Check sheet for the modelled part. Datum: model origin and axes. Units: mm. A direction names the side the tool comes from. Coordinates: 2 decimals unless noted, no trailing zeros. Loops run counter-clockwise (first coordinate to the right, second up) from the corner with the lowest first, then second, coordinate; pieces in that order, holes last. Notation, with made-up numbers: (84.25, -35.5) - (96.25, -35.5) arc R5 cw to (96.25, -30.5) - close; hole circle Ø3 at (40.25, -8). An arc over 180 degrees is marked (long way). Use a Markdown table: item, result. Add a question column.
1) Tool access check on faces 1 (the flat face through (-4, 16, 4)), 2 (the flat face through (6, 6.29, -2)), 3 (the flat face through (-3.537, 16.247, -3.484)), 4 (the flat face through (-4.24, 16.25, -2.71)). Record the directions out of +Z, -Z, +X, -X, +Y, -Y that give a thin tool (end or side, any length) a straight path to the whole face; none if there is none.
2) Go/stop test with flat-tipped pins: P1, Ø1.5, axis at x = -3, z = -6, coming from the +Y side; P2, Ø3, axis at y = 11, z = -1.5, coming from the +X side; P3, Ø2, axis at x = 3.5, y = 9, coming from the -Z side. Record where each tip stops, or that it passes through.
3) Sectioned sample at A-A, the plane z = 0. Enter the section's corners in (x, y).
4) Thickness scan on line 1 (Y direction, x = 5.75, z = 4); line 2 (X direction, y = 4.75, z = 0); line 3 (X direction, y = 7, z = 0). Record the ranges inside material, lowest first.
5) Sectioned sample at B-B, the plane y = 7. Enter the section's corners in (x, z).
6) Draft check along Z on faces 5 (the flat face through (-4.765, 16.247, 1.627)), 6 (the flat face through (0, 0, 3)), 7 (the cylindrical face through (1.802, 10.234, 5.723)). Enter one of: pulls with the +Z half, pulls with the -Z half, needs draft (parallel to the pull), parting line crosses it, or undercut.
from build123d import *
from build123d.topology import SkipClean

# Parameters (mm, degrees)
SKETCH2_R           = 7.5
SKETCH2_R_2         = 2.5
BOSS_EXTRUDE1_DEPTH = 16
SKETCH3_OUTSIDE_W   = 22.314
SKETCH3_OUTSIDE_H   = 22.314
SKETCH3_OUTSIDE_R   = 6
CUT_EXTRUDE1_DEPTH  = 8
CHAMFER1_SIZE       = 0.5
BOSS_EXTRUDE2_DEPTH = 0.5


with BuildPart() as part:
    # Sketch2 → Boss-Extrude1 (new body)
    with BuildSketch(Plane(origin=(0, 0, 0), x_dir=(1, 0, 0), z_dir=(0, 1, 0))):
        with Locations(Location((0, 0, 0), (0, 0, 270))):
            Circle(SKETCH2_R)
        with Locations(Location((0, 0, 0), (0, 0, 270))):
            Circle(SKETCH2_R_2, mode=Mode.SUBTRACT)
    extrude(amount=BOSS_EXTRUDE1_DEPTH)

    # Sketch3 outside → Cut-Extrude1 (cut)
    with BuildSketch(Plane(origin=(0, 6.29, 0), x_dir=(1, 0, 0), z_dir=(0, 1, 0))):
        Rectangle(SKETCH3_OUTSIDE_W, SKETCH3_OUTSIDE_H)
        with Locations(Location((0, 0, 0), (0, 0, 270))):
            Circle(SKETCH3_OUTSIDE_R, mode=Mode.SUBTRACT)
    extrude(amount=CUT_EXTRUDE1_DEPTH, mode=Mode.SUBTRACT)

    # Chamfer1
    chamfer1_edges = [part.edges().sort_by_distance(p)[0] for p in [
        (0, 6.29, -7.5),
        (0, 0, -7.5),
    ]]
    chamfer(chamfer1_edges, length=CHAMFER1_SIZE)

    # Sketch7 → Boss-Extrude2 (add)
    with SkipClean():  # the faces are left unmerged after this step: merging them gives an invalid solid
        with BuildSketch(Plane(origin=(0, 16, 0), x_dir=(1, 0, 0), z_dir=(0, 1, 0))):
            with BuildLine():
                ThreePointArc((0.783963475, 7.458914215), (0.392519672, 7.489721511), (0, 7.5))
                Line((0, 7.5), (0, 2.5))
                ThreePointArc((0, 2.5), (0.130839891, 2.496573837), (0.261321158, 2.486304738))
                Line((0.261321158, 2.486304738), (0.783963475, 7.458914215))
            make_face()
            with BuildLine():
                Line((0, 2.5), (0, 7.5))
                ThreePointArc((0, 7.5), (-0.392519672, 7.489721511), (-0.783963475, 7.458914215))
                Line((-0.783963475, 7.458914215), (-0.261321158, 2.486304738))
                ThreePointArc((-0.261321158, 2.486304738), (-0.130839891, 2.496573837), (0, 2.5))
            make_face()
            with BuildLine():
                Line((-1.780940242, 1.754494757), (-5.342820727, 5.263484272))
                ThreePointArc((-5.342820727, 5.263484272), (-5.863736119, 4.676173514), (-6.32040719, 4.037629621))
                Line((-6.32040719, 4.037629621), (-2.106802397, 1.34587654))
                ThreePointArc((-2.106802397, 1.34587654), (-1.954578706, 1.558724505), (-1.780940242, 1.754494757))
            make_face()
            with BuildLine():
                Line((-2.482117316, -0.298485561), (-7.446351948, -0.895456684))
                ThreePointArc((-7.446351948, -0.895456684), (-7.311959341, -1.668907005), (-7.097455378, -2.424072431))
                Line((-7.097455378, -2.424072431), (-2.365818459, -0.808024144))
                ThreePointArc((-2.365818459, -0.808024144), (-2.43731978, -0.556302335), (-2.482117316, -0.298485561))
            make_face()
            with BuildLine():
                Line((-1.314209425, -2.126700164), (-3.942628274, -6.380100493))
                ThreePointArc((-3.942628274, -6.380100493), (-3.254128043, -6.757266509), (-2.529974905, -7.0603985))
                Line((-2.529974905, -7.0603985), (-0.843324968, -2.353466167))
                ThreePointArc((-0.843324968, -2.353466167), (-1.084709348, -2.25242217), (-1.314209425, -2.126700164))
            make_face()
            with BuildLine():
                ThreePointArc((2.529974905, -7.0603985), (3.254128043, -6.757266509), (3.942628274, -6.380100493))
                Line((3.942628274, -6.380100493), (1.314209425, -2.126700164))
                ThreePointArc((1.314209425, -2.126700164), (1.084709348, -2.25242217), (0.843324968, -2.353466167))
                Line((0.843324968, -2.353466167), (2.529974905, -7.0603985))
            make_face()
            with BuildLine():
                ThreePointArc((7.097455378, -2.424072431), (7.311959341, -1.668907005), (7.446351948, -0.895456684))
                Line((7.446351948, -0.895456684), (2.482117316, -0.298485561))
                ThreePointArc((2.482117316, -0.298485561), (2.43731978, -0.556302335), (2.365818459, -0.808024144))
                Line((2.365818459, -0.808024144), (7.097455378, -2.424072431))
            make_face()
            with BuildLine():
                ThreePointArc((6.32040719, 4.037629621), (5.863736119, 4.676173514), (5.342820727, 5.263484272))
                Line((5.342820727, 5.263484272), (1.780940242, 1.754494757))
                ThreePointArc((1.780940242, 1.754494757), (1.954578706, 1.558724505), (2.106802397, 1.34587654))
                Line((2.106802397, 1.34587654), (6.32040719, 4.037629621))
            make_face()
        extrude(amount=BOSS_EXTRUDE2_DEPTH)


solid = part.part
Solved:
| question | item | result |
|---|---|---|
| 1 | face 1 | +Y |
| 1 | face 2 | none |
| 1 | face 3 | -Z, +Y |
| 1 | face 4 | -X, +Y |
| 2 | P1 | stops at y = 16 |
| 2 | P2 | stops at x = 6 |
| 2 | P3 | stops at z = -5.45 |
| 3 | outline | (-7.5, 0.5) - (-7, 0) - (-2.5, 0) - (-2.5, 16) - (-7.5, 16) - (-7.5, 14.29) - (-6, 14.29) - (-6, 6.29) - (-7, 6.29) - (-7.5, 5.79) - close; (2.5, 0) - (7, 0) - (7.5, 0.5) - (7.5, 5.79) - (7, 6.29) - (6, 6.29) - (6, 14.29) - (7.5, 14.29) - (7.5, 16) - (2.5, 16) - close |
| 4 | line 1 | y = 0 to 6.29, 14.29 to 16 |
| 4 | line 2 | x = -7.5 to -2.5, 2.5 to 7.5 |
| 4 | line 3 | x = -6 to -2.5, 2.5 to 6 |
| 5 | outline | circle Ø12 at (0, 0); hole circle Ø5 at (0, 0) |
| 6 | face 5 | undercut |
| 6 | face 6 | needs draft |
| 6 | face 7 | parting line crosses it |
